Read the model definition and answer for the solid it produces. Units are mm, in the model's axes. A direction names the side the tool comes from. Round coordinates to 2 decimals unless told otherwise and drop trailing zeros. Write each loop counter-clockwise with the first axis right and the second up, starting at its lowest first coordinate (ties: lowest second). Pieces come first, ordered by that corner, then holes. Notation, with made-up numbers: (-10, 46.25) -> (5, 46.25) arc R19 cw to (5, 71.25) -> close; hole circle Ø8 at (-14.5, 69). An arc over 180 degrees is marked (long way). Return JSON: item names as keys, results as strings.
from build123d import *

# Parameters (mm, degrees)
SKETCH_1_R               = 6.45
EXTRUDE_1_DEPTH          = 43
CUT_EXTRUDE_3_DEPTH      = 92.963760979
SKETCH_3_R               = 2.125
CUT_EXTRUDE_4_DEPTH      = 15
PATTERN_CIRCULAR_1_COUNT = 3
SKETCH_4_R               = 2.125
CUT_EXTRUDE_5_DEPTH      = 118.823314048
SKETCH_6_R               = 2.15
CUT_EXTRUDE_7_DEPTH      = 128.471565491
SKETCH_7_R               = 4.5
CUT_EXTRUDE_8_DEPTH      = 15


with BuildPart() as part:
    # 草图1 → 凸台-拉伸1 (new body)
    with BuildSketch(Plane.XY):
        Polygon((5.773502692, 60), (-5.773502692, 60), (-54.848275573, -25), (-49.074772881, -35), (49.074772881, -35), (54.848275573, -25), align=None)
        Circle(SKETCH_1_R, mode=Mode.SUBTRACT)
    extrude(amount=EXTRUDE_1_DEPTH)

    # 草图2 → 切除-拉伸3 (cut, through all)
    with BuildSketch(Plane.XY.offset(43)):
        Polygon((5.759618943, 39.975952642), (0, 43.301270189), (-5.759618943, 39.975952642), (0, 30), align=None)
        Polygon((0, 43.301270189), (-2.900635095, 44.975952642), (-11.650635095, 29.820508076), (-2.990381057, 24.820508076), (0, 30), (-5.759618943, 39.975952642), align=None)
        Polygon((2.900635095, 44.975952642), (0, 43.301270189), (5.759618943, 39.975952642), (0, 30), (2.990381057, 24.820508076), (11.650635095, 29.820508076), align=None)
        Polygon((-22.990381057, -9.820508076), (-31.650635095, -4.820508076), (-40.400635095, -19.975952642), (-37.5, -21.650635095), (-37.5, -15), (-25.980762114, -15), align=None)
        Polygon((-37.5, -15), (-37.5, -21.650635095), (-31.740381057, -24.975952642), (-25.980762114, -15), align=None)
        Polygon((-31.740381057, -24.975952642), (-37.5, -21.650635095), (-37.5, -25), (-20, -25), (-20, -15), (-25.980762114, -15), align=None)
        Polygon((25.980762114, -15), (20, -15), (20, -25), (37.5, -25), (37.5, -21.650635095), (31.740381057, -24.975952642), align=None)
        Polygon((37.5, -15), (25.980762114, -15), (31.740381057, -24.975952642), (37.5, -21.650635095), align=None)
        Polygon((40.400635095, -19.975952642), (31.650635095, -4.820508076), (22.990381057, -9.820508076), (25.980762114, -15), (37.5, -15), (37.5, -21.650635095), align=None)
        Polygon((2.900635095, 44.975952642), (-2.900635095, 44.975952642), (0, 43.301270189), align=None)
        Polygon((-37.5, -21.650635095), (-40.400635095, -19.975952642), (-37.5, -25), align=None)
        Polygon((37.5, -25), (40.400635095, -19.975952642), (37.5, -21.650635095), align=None)
        Polygon((25.980762114, -15), (22.990381057, -9.820508076), (20, -15), align=None)
        Polygon((-20, -15), (-22.990381057, -9.820508076), (-25.980762114, -15), align=None)
        Polygon((0, 30), (-2.990381057, 24.820508076), (2.990381057, 24.820508076), align=None)
    extrude(amount=-CUT_EXTRUDE_3_DEPTH, mode=Mode.SUBTRACT)

    # 草图3 → 切除-拉伸4 (cut)
    with BuildSketch(Plane(origin=(-30.310889132, 17.5, 0), x_dir=(0, 0, 1), z_dir=(-0.8660254037844362, 0.5000000000000046, 0))):
        with Locations(Location((21.5, 28, 0), (0, 0, 270))):
            Circle(SKETCH_3_R)
        with Locations(Location((21.5, -28, 0), (0, 0, 90))):
            Circle(SKETCH_3_R)
    cut_extrude_4 = extrude(amount=-CUT_EXTRUDE_4_DEPTH, mode=Mode.SUBTRACT)

    # 阵列(圆周)1: 切除-拉伸4 ×3 about axis
    pattern_circular_1_axis = Axis((0, 0, 43), (0, 0, -1))
    for i in range(1, PATTERN_CIRCULAR_1_COUNT):
        add(cut_extrude_4.rotate(pattern_circular_1_axis, i * 360 / PATTERN_CIRCULAR_1_COUNT), mode=Mode.SUBTRACT)

    # 草图4 → 切除-拉伸5 (cut, through all)
    with BuildSketch(Plane.XZ.offset(35)):
        with Locations(Location((0, 13, 0), (0, 0, 270))):
            Circle(SKETCH_4_R)
        with Locations(Location((0, 28, 0), (0, 0, 270))):
            Circle(SKETCH_4_R)
    extrude(amount=-CUT_EXTRUDE_5_DEPTH, mode=Mode.SUBTRACT)

    # 草图6 → 切除-拉伸7 (cut, through all)
    with BuildSketch(Plane(origin=(49.074772881, 0, 0), x_dir=(0, 0, -1), z_dir=(-1, 0, 0))):
        with Locations(Location((-23, 0, 0), (0, 0, 270))):
            Circle(SKETCH_6_R)
        with Locations(Location((-38, 0, 0), (0, 0, 270))):
            Circle(SKETCH_6_R)
    extrude(amount=CUT_EXTRUDE_7_DEPTH, mode=Mode.SUBTRACT)

    # 草图7 → 切除-拉伸8 (cut)
    with BuildSketch(Plane(origin=(49.074772881, 0, 0), x_dir=(0, 0, -1), z_dir=(-1, 0, 0))):
        with Locations(Location((-38, 0, 0), (0, 0, 90))):
            Circle(SKETCH_7_R)
        with Locations(Location((-23, 0, 0), (0, 0, 90))):
            Circle(SKETCH_7_R)
    extrude(amount=CUT_EXTRUDE_8_DEPTH, mode=Mode.SUBTRACT)


solid = part.part
Item 1: For a pull along Y with two mould halves and no side action, classify faces 4 (the flat face through (-36.94, -13.98, 21.8)), 5 (the flat face through (20, -20, 22)), 6 (the flat face through (51.92, -30.07, 21.2)), 7 (the cylindrical face through (-29.69, -30.07, 20.21)) as released by +Y, released by -Y, zero draft, split by the parting line, or undercut.
Worked answers:
{"face 4": "undercut", "face 5": "undercut", "face 6": "released by -Y", "face 7": "zero draft"}
Item 2: Section B-B (z = 13) is taken. State how many separate pieces and enclosed holes the cut face has, then the cut area to 3 significant figures.
Worked answers:
{"separate pieces": "2", "enclosed holes": "2", "area": "4,920 mm2"}
Item 3: Flat-ended cylindrical pins translate along their axes: pin 1 (9 mm diameter, centred on x = -31, z = 16.5, fed in from +Y); pin 2 (1.5 mm diameter, centred on y = 44.5, z = 5, fed in from -X); pin 3 (8 mm diameter, centred on y = 44, z = 35, fed in from +X). Find the tip coordinate at first contact, or state that the pin passes through.
Worked answers:
{"pin 1": "stops at y = 24.1", "pin 2": "stops at x = -15.16", "pin 3": "stops at x = 17.32"}
Item 4: Straight lines are drawn through the part: L1, parallel to Z at x = 23.75, y = 0; L2, parallel to Z at x = 37, y = 0; L3, parallel to Y at x = 38.5, z = 41.5. For each, find the intervals that lie inside material, in ascending order. Write a range as [from, to].
Worked answers:
{"L1": "z = [0, 20.85], [25.15, 35.85], [40.15, 43]", "L2": "z = [0, 18.5], [27.5, 33.5], [42.5, 43]", "L3": "y = [-35, -23.27], [-16.68, -2.83], [2.83, 3.32]"}
Item 5: Section A-A (x = -28) is taken. Give the vertices of the cut face in (y, z) (3 decimals), then the cut area to 3 significant figures.
Worked answers:
{"outline": "(-35, 0) -> (-25, 0) -> (-25, 19.375) -> (-35, 19.375) -> close; (-35, 23.625) -> (-25, 23.625) -> (-25, 43) -> (-35, 43) -> close; (-6.928, 0) -> (21.503, 0) -> (21.503, 43) -> (-6.928, 43) -> close; hole circle Ø4.3 at (0, 23); hole circle Ø4.3 at (0, 38)", "area": "1,580 mm2"}
Item 6: Section C-C (y = -22) is taken. Give the vertices of the cut face in (x, z) (3 decimals), then the cut area to 3 significant figures.
Worked answers:
{"outline": "(-53.116, 0) -> (-39.232, 0) -> (-39.232, 43) -> (-53.116, 43) -> close; (-20, 0) -> (20, 0) -> (20, 43) -> (-20, 43) -> close; (39.232, 0) -> (53.116, 0) -> (53.116, 43) -> (39.232, 43) -> close; hole circle Ø4.25 at (0, 13); hole circle Ø4.25 at (0, 28)", "area": "2,890 mm2"}
Item 7: A tool of negligible diameter and unlimited length cuts with its end or side. For faces 1 (the cylindrical face through (20.27, -0.28, 35.87)), 2 (the flat face through (31, -25, 22)), 3 (the cylindrical face through (37.613, -4.292, 24.352)), from which of +Z, -Z, +X, -X, +Y, -Y can it reach the whole face along a straight path? Write none if from no direction.
Worked answers:
{"face 1": "+X, -X", "face 2": "+Z, -Z", "face 3": "+X"}
